For this review, take the finished solid that the model builds, in its own axes (mm). A direction names the side the tool comes from. Give positions to 0.01 mm unless a question says otherwise; leave off trailing zeros. Loops run counter-clockwise (first coordinate to the right, second up) from the corner with the lowest first, then second, coordinate; pieces in that order, holes last. Notation, with made-up numbers: (79.5, -29) - (116.5, -29) arc R22 cw to (116.5, -4) - close; hole circle Ø5 at (67.25, -26.5). An arc over 180 degrees is marked (long way). Put each result on its own line as item: value.
from build123d import *

# Parameters (mm, degrees)
F0_R     = 3.55
F1_DEPTH = 3.86
F3_DEPTH = 2.5
F4_R     = 2
F5_DEPTH = 12
F6_SIZE  = 0.5


with BuildPart() as f1:
    # F0 (on Front) → F1 (new body)
    with BuildSketch(Plane.XZ):
        Circle(F0_R)
    extrude(amount=F1_DEPTH)

    # F2 (on face) → F3 (cut)
    with BuildSketch(Plane.XZ.offset(3.86)):
        Polygon((-1.030145, -1.784263), (1.030145, -1.784263), (2.060289, 0), (1.030145, 1.784263), (-1.030145, 1.784263), (-2.060289, 0), align=None)
    extrude(amount=-F3_DEPTH, mode=Mode.SUBTRACT)

    # F4 (on face) → F5 (join)
    with BuildSketch(Plane(origin=(0, 0, 0), x_dir=(-1, 0, 0), z_dir=(0, 1, 0))):
        Circle(F4_R)
    extrude(amount=F5_DEPTH)

    # F6
    f6_edges = [f1.edges().sort_by_distance(p)[0] for p in [
        (-3.55, -3.86, 0),
    ]]
    chamfer(f6_edges, length=F6_SIZE)


solid = f1.part
1) Take a section at B-B on y = -0.25. State the section outline as (x, z) points.
Geometry check:
outline: circle Ø7.1 at (0, 0)
2) Take a section at A-A on x = 0. State the section outline as (y, z) points, and give its area (3 significant figures).
Geometry check:
outline: (-3.86, -3.05) - (-3.36, -3.55) - (0, -3.55) - (0, -2) - (12, -2) - (12, 2) - (0, 2) - (0, 3.55) - (-3.36, 3.55) - (-3.86, 3.05) - (-3.86, 1.78) - (-1.36, 1.78) - (-1.36, -1.78) - (-3.86, -1.78) - close
area: 66.2 mm²
3) Wall thickness on line 1 (Y direction, x = -1, z = 1); line 2 (Z direction, x = 0, y = 5.25); line 3 (Z direction, x = -0.5, y = -1.5): over which ranges is each line inside the solid? List them lowest first.
Geometry check:
line 1: y = -1.36 to 12
line 2: z = -2 to 2
line 3: z = -3.51 to -1.78, 1.78 to 3.51
4) Insertion check: pin 1 Ø1.1 at (x, z) = (0.5, 0) entering from -Y; pin 2 Ø3 at (y, z) = (2.5, 0.5) entering from -X; pin 3 Ø1 at (y, z) = (-1, -2) entering from +X. Each pin has a flat end and moves straight along its axis. Give the tip position at first contact, or say it passes through.
Geometry check:
pin 1: stops at y = -1.36
pin 2: stops at x = -2
pin 3: stops at x = 3.22
5) Take a section at C-C on y = 8.75. State the section outline as (x, z) points.
Geometry check:
outline: circle Ø4 at (0, 0)
6) For faces 5 (the face through (2, 0, -2)), 6 (the face through (0, -1.36, 0)), 7 (the face through (-0.46, -1.66, 3.52)), list the 3-axis set-ups (+Z, -Z, +X, -X, +Y, -Y) from which the entire face can be reached by the end or side of a thin tool; tool diameter is ignored.
Geometry check:
face 5: +Y
face 6: -Y
face 7: +Y, -Y
7) Draft analysis for pull direction Z (two halves, no side actions). For faces 1 (the face through (0, 6, -2)), 2 (the face through (1.54, -2.63, -0.9)), 3 (the face through (0, -3, -1.784)), 4 (the face through (0, 12, 0)), state which applies: pulls with the +Z half, pulls with the -Z half, needs draft (parallel to the pull), parting line crosses it, or undercut.
Geometry check:
face 1: parting line crosses it
face 2: undercut
face 3: undercut
face 4: needs draft
